Input: dimensioned drawing with shaded views. Units: mm. Origin: part minimum x, y, z. Coordinates: 2 decimals unless noted, no trailing zeros. Order: outer loops, then holes, each group sorted by start corner. A loop starts at its lowest first (then second) coordinate and runs counter-clockwise, first axis right, second up.
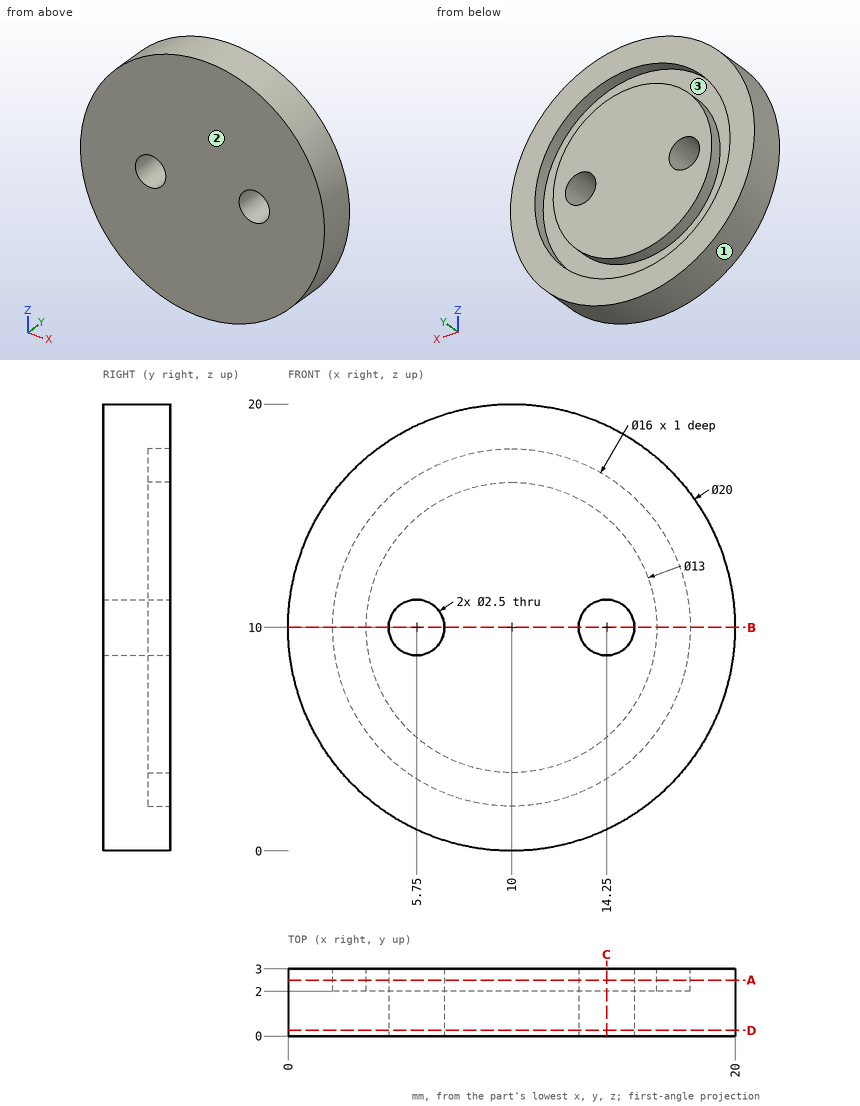
1. Section query A-A on y = 2.5. Return loops of the section in (x, z), plus the area to 3 significant figures.
Findings:
outline: circle Ø20 at (10, 10); circle Ø13 at (10, 10); hole circle Ø16 at (10, 10); hole circle Ø2.5 at (5.75, 10); hole circle Ø2.5 at (14.25, 10)
area: 236 mm2
2. Pin query (flat end, axial travel): P1, Ø2, axis at x = 5.75, z = 10, coming from the +Y side; P2, Ø1, axis at x = 4.5, y = 1, coming from the -Z side. Return the tip coordinate at first contact, or that it passes through.
Findings:
P1: passes through
P2: stops at z = 1.34
3. Section query D-D on y = 0.25. Return loops of the section in (x, z), plus the area to 3 significant figures.
Findings:
outline: circle Ø20 at (10, 10); hole circle Ø2.5 at (5.75, 10); hole circle Ø2.5 at (14.25, 10)
area: 304 mm2
4. Section query C-C on x = 14.25. Return loops of the section in (y, z), plus the area to 3 significant figures.
Findings:
outline: (0, 0.95) - (3, 0.95) - (3, 3.22) - (2, 3.22) - (2, 5.08) - (3, 5.08) - (3, 8.75) - (0, 8.75) - close; (0, 11.25) - (3, 11.25) - (3, 14.92) - (2, 14.92) - (2, 16.78) - (3, 16.78) - (3, 19.05) - (0, 19.05) - close
area: 43.1 mm2
5. Section query B-B on z = 10. Return loops of the section in (x, y), plus the area to 3 significant figures.
Findings:
outline: (0, 0) - (4.5, 0) - (4.5, 3) - (3.5, 3) - (3.5, 2) - (2, 2) - (2, 3) - (0, 3) - close; (7, 0) - (13, 0) - (13, 3) - (7, 3) - close; (15.5, 0) - (20, 0) - (20, 3) - (18, 3) - (18, 2) - (16.5, 2) - (16.5, 3) - (15.5, 3) - close
area: 42.0 mm2
6. Ray query, line 1 (X direction, y = 2.35, z = 10); line 2 (X direction, y = 1.05, z = 10); line 3 (Z direction, x = 6, y = 2.7). Return the intervals inside material, ascending.
Findings:
line 1: x = 0 to 2, 3.5 to 4.5, 7 to 13, 15.5 to 16.5, 18 to 20
line 2: x = 0 to 4.5, 7 to 13, 15.5 to 20
line 3: z = 0.83 to 3.07, 4.88 to 8.78, 11.22 to 15.12, 16.93 to 19.17
7. Draft query along Z for the marked faces 1, 2 and 3. Return one class per face: released by +Z, released by -Z, zero draft, split by the parting line, or undercut.
Findings:
face 1: split by the parting line
face 2: zero draft
face 3: undercut
